Model file for the job. Use its own axes, mm. A direction names the side the tool comes from. Round coordinates to 2 decimals unless told otherwise and drop trailing zeros. Order: outer loops, then holes, each group sorted by start corner. A loop starts at its lowest first (then second) coordinate and runs counter-clockwise, first axis right, second up. Notation, with made-up numbers: (3.5, -21.75) - (28.5, -21.75) arc R35 ccw to (28.5, 15.25) - close; hole circle Ø10 at (48, 58). An arc over 180 degrees is marked (long way). Write item = value, one per line.
Solid Edge part; units mm, degrees
sketch "Sketch1" plane through (0, 0, 0) normal (0, -1, 0) x (1, 0, 0)
  line L0 (-20.5, 20) -> (13.5, 20)
  line L1 (13.5, 20) -> (20.5, 16)
  line L2 (20.5, 16) -> (20.5, -20)
  line L3 (20.5, -20) -> (-20.5, -20)
  line L4 (-20.5, -20) -> (-20.5, 20)
extrude "Protrusion1" add sketch "Sketch1" along normal mid plane 20.2
sketch "Sketch2" plane through (3.5, -10.1, 0) normal (0, -1, 0) x (1, 0, 0)
  line L0 (17, 11.5) -> (24.5, 11.5)
  line L1 (24.5, 11.5) -> (24.5, 9)
  line L2 (17, 9) -> (24.5, 9)
  line L3 (17, 11.5) -> (17, 9)
extrude "Protrusion2" add sketch "Sketch2" against normal up to vertex (20.2 mm away)
mirror "Mirror1" about plane through (0, 0, 0) normal (1, 0, 0) of "Protrusion2"
sketch "Sketch3" plane through (-3.5, 0, 20) normal (0, 0, 1) x (0, 1, 0)
  circle A0 centre (0, 6.5) radius 6.5
sketch "Sketch4" plane through (-3.5, 0, 22) normal (0, 0, 1) x (1, 0, 0)
  circle A0 centre (-6.5, 0) radius 5.5
loft "LoftedProtrusion1" add profiles "Sketch3", "Sketch4"
sketch "Sketch5" plane through (-13.5, 0, 22) normal (0, 0, 1) x (1, 0, 0)
  circle A0 centre (3.5, 0) radius 3
extrude "ProtrusiónExtruida_4" add sketch "Sketch5" along normal blind 4
sketch "Sketch6" plane through (-27.75, 0, 11.5) normal (0, 0, 1) x (1, 0, 0)
  circle A0 centre (2.35, 5.6) radius 2.5
extrude "Cutout1" cut sketch "Sketch6" against normal up to vertex (2.5 mm away)
mirror "Mirror2" about plane through (0, 0, 0) normal (0, -1, 0) of "Cutout1"
mirror "Mirror3" about plane through (0, 0, 0) normal (1, 0, 0) of "Cutout1", "Mirror2"
sketch "Sketch7" plane through (-3.5, 0, 20) normal (0, 0, 1) x (0, 1, 0)
  line L0 (10.1, 4) -> (8.1, 4)
  line L1 (8.1, 4) -> (8.1, 9)
  line L2 (8.1, 9) -> (10.1, 9)
  line L3 (10.1, 9) -> (10.1, 4)
extrude "ProtrusiónExtruida_5" add sketch "Sketch7" along normal blind 1
mirror "Mirror4" about plane through (0, 0, 0) normal (0, -1, 0) of "ProtrusiónExtruida_5"
hole "Agujero_2" at (-10, 0, 26) direction (0, 0, -1) diameter 3 depth 8
1) Cut at B-B (y = 0). Write the cut outline in (x, z).
Conclusion:
outline = (-28, 9) - (-20.5, 9) - (-20.5, -20) - (20.5, -20) - (20.5, 9) - (28, 9) - (28, 11.5) - (20.5, 11.5) - (20.5, 16) - (13.5, 20) - (-3.5, 20) - (-4.5, 22) - (-7, 22) - (-7, 26) - (-8.5, 26) - (-8.5, 18) - (-11.5, 18) - (-11.5, 26) - (-13, 26) - (-13, 22) - (-15.5, 22) - (-16.5, 20) - (-20.5, 20) - (-20.5, 11.5) - (-28, 11.5) - close
2) Wall check: line 1 along Z through (x, y) = (24.5, 2.5); line 2 along X through (y, z) = (-4, -0.5); line 3 along Z through (x, y) = (-8, -3.75). Give the ranges that are in metal, low to high.
Conclusion:
line_1 = 9 to 11.5
line_2 = -20.5 to 20.5
line_3 = -20 to 22
3) Mould opens along X. For faces 5 (the face through (-20.5, 0, -6)), 6 (the face through (24.06, -7.71, 10.27)), 7 (the face through (20.5, 0, -5)) say: +X half, -X half, draft (parallel to the pull), parting line (faces both ways), or undercut.
Conclusion:
face_5 = -X half
face_6 = undercut
face_7 = +X half
4) Flat gauge pins, fed straight in: pin 1 Ø5 at (x, y) = (9.5, -2.5) entering from +Z; pin 2 Ø4 at (x, y) = (23.5, -3.5) entering from +Z; pin 3 Ø0.5 at (y, z) = (9, 20.5) entering from -X. Where does each tip first touch, or does it go through?
Conclusion:
pin_1 = 20
pin_2 = 11.5
pin_3 = -12.5
5) 3-axis set-ups, long thin cutter, end or side, ignore diameter. For faces 1 (the face through (-24, 0, 9)), 2 (the face through (20.5, 0, 14)), 3 (the face through (-24, 0, 11.5)), 4 (the face through (-8.536, 0.325, 21.944)): which of +Z, -Z, +X, -X, +Y, -Y reach the whole face in a straight line?
Conclusion:
face_1 = -Z, -X, +Y, -Y
face_2 = +Z, +X, +Y, -Y
face_3 = +Z, -X, +Y, -Y
face_4 = +Z
6) Cut at A-A (x = -25.4). Write the cut outline in (y, z), and give its area (3 significant figures).
Conclusion:
outline = (-10.1, 9) - (-8.1, 9) - (-8.1, 11.5) - (-10.1, 11.5) - close; (-3.1, 9) - (3.1, 9) - (3.1, 11.5) - (-3.1, 11.5) - close; (8.1, 9) - (10.1, 9) - (10.1, 11.5) - (8.1, 11.5) - close
area = 25.5 mm^2
7) Cut at C-C (x = -17.5). Write the cut outline in (y, z), and give its area (3 significant figures).
Conclusion:
outline = (-10.1, -20) - (10.1, -20) - (10.1, 20) - (-10.1, 20) - close
area = 808 mm^2
8) Cut at D-D (y = 4). Give the number of separate pieces and of enclosed holes in the cut face, and give its area (3 significant figures).
Conclusion:
separate_pieces = 3
enclosed_holes = 0
area = 1,660 mm^2
